from build123d import *

# Parameters (mm, degrees)
SKETCH2_W           = 12.25
SKETCH2_H           = 4
BOSS_EXTRUDE1_DEPTH = 10
SKETCH3_R           = 0.5
CUT_EXTRUDE1_DEPTH  = 5


with BuildPart() as part:
    # Sketch2 → Boss-Extrude1 (new body)
    with BuildSketch(Plane.XY):
        with Locations((6.125, 2)):
            Rectangle(SKETCH2_W, SKETCH2_H)
    extrude(amount=BOSS_EXTRUDE1_DEPTH)

    # Sketch3 → Cut-Extrude1 (cut)
    with BuildSketch(Plane.XY.offset(10)):
        with Locations((1.125, 2)):
            Circle(SKETCH3_R)
        with Locations((2.375, 2)):
            Circle(SKETCH3_R)
        with Locations((3.625, 2)):
            Circle(SKETCH3_R)
        with Locations((4.875, 2)):
            Circle(SKETCH3_R)
        with Locations((6.125, 2)):
            Circle(SKETCH3_R)
        with Locations((7.375, 2)):
            Circle(SKETCH3_R)
        with Locations((8.625, 2)):
            Circle(SKETCH3_R)
        with Locations((9.875, 2)):
            Circle(SKETCH3_R)
        with Locations((11.125, 2)):
            Circle(SKETCH3_R)
    extrude(amount=-CUT_EXTRUDE1_DEPTH, mode=Mode.SUBTRACT)


solid = part.part
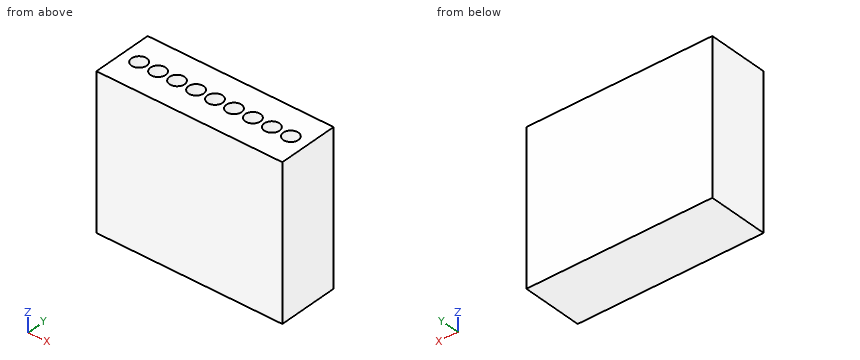
Model file for the job. Use its own axes, mm. Give positions to 0.01 mm unless a question says otherwise; leave off trailing zeros. Loops run counter-clockwise (first coordinate to the right, second up) from the corner with the lowest first, then second, coordinate; pieces in that order, holes last.
1) Flat gauge pin, fed straight in: pin 1 Ø0.5 at (x, y) = (2.5, 2) entering from +Z. Where does the tip first touch, or does it go through?
2) Wall check: line 1 (Y direction, x = 11, z = 8.5); line 2 (Y direction, x = 1.5, z = 7.5). Give the ranges that are in metal, low to high.
3) Saw through at B-B (x = 5). Write the cut outline in (y, z), plus the area to 3 significant figures.
4) Saw through at A-A (z = 9). Count the separate pieces of the cut face and the enclosed holes in it, plus the area to 3 significant figures.
Answer block:
1. pin 1: stops at z = 5
2. line 1: y = 0 to 1.52, 2.48 to 4
2. line 2: y = 0 to 1.67, 2.33 to 4
3. outline: (0, 0) - (4, 0) - (4, 10) - (2.48, 10) - (2.48, 5) - (1.52, 5) - (1.52, 10) - (0, 10) - close
3. area: 35.2 mm2
4. separate pieces: 1
4. enclosed holes: 9
4. area: 41.9 mm2
